The listing builds one solid part. Answer for the finished solid, in the listing's coordinates (mm). Face numbers are marked on the shaded views. A direction names the side the tool comes from. Round coordinates to 2 decimals unless told otherwise and drop trailing zeros. Loops run counter-clockwise (first coordinate to the right, second up) from the corner with the lowest first, then second, coordinate; pieces in that order, holes last. Notation, with made-up numbers: (-24.75, 5.25) -> (12.25, 5.25) arc R38 ccw to (12.25, 43.25) -> close; hole circle Ø6 at (47, -35). An arc over 180 degrees is marked (long way). One line per question, with ' | ' between items.
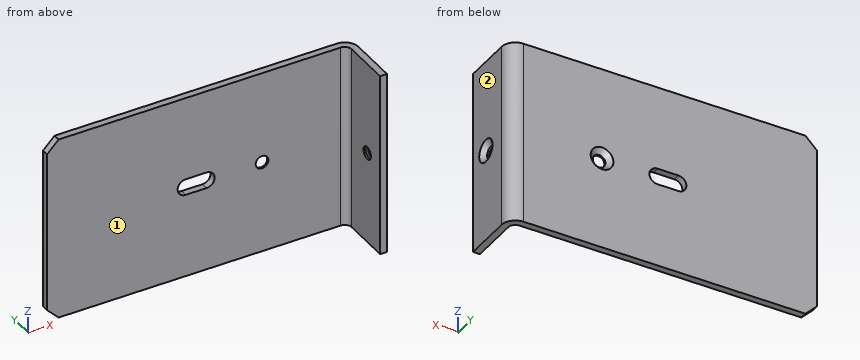
from build123d import *

# Parameters (mm, degrees)
BASE_EXTRU_MINCE_DEPTH  = 40
CHANFREIN1_SIZE         = 5
ESQUISSE3_R             = 2.75
ENL_V_MAT_EXTRU_1_DEPTH = 139.668669857
ESQUISSE4_R             = 2.75
ENL_V_MAT_EXTRU_2_DEPTH = 141.943250991
CHANFREIN2_SIZE         = 2.15


with BuildPart() as part:
    # Esquisse1 → Base-Extru.-Mince (new, symmetric)
    with BuildSketch(Plane.XY):
        with BuildLine():
            Line((0, -24), (0, -3))
            ThreePointArc((0, -3), (-0.878679656, -0.878679656), (-3, 0))
            Line((-3, 0), (-130, 0))
            Line((-130, 0), (-130, 3))
            Line((-130, 3), (-3, 3))
            ThreePointArc((-3, 3), (1.242640687, 1.242640687), (3, -3))
            Line((3, -3), (3, -24))
            Line((3, -24), (0, -24))
        make_face()
    extrude(amount=BASE_EXTRU_MINCE_DEPTH, both=True)

    # Chanfrein1
    chanfrein1_edges = [part.edges().sort_by_distance(p)[0] for p in [
        (-130, 1.5, 40),
        (-130, 1.5, -40),
    ]]
    chamfer(chanfrein1_edges, length=CHANFREIN1_SIZE)

    # Esquisse3 → Enl_v. mat.-Extru.1 (cut, through all)
    with BuildSketch(Plane(origin=(0, 3, 0), x_dir=(-1, 0, 0), z_dir=(0, 1, 0))):
        with Locations((37, 0)):
            Circle(ESQUISSE3_R)
        with BuildLine():
            Line((70, 3.5), (61, 3.5))
            ThreePointArc((61, 3.5), (57.5, 0), (61, -3.5))
            Line((61, -3.5), (70, -3.5))
            ThreePointArc((70, -3.5), (73.5, 0), (70, 3.5))
        make_face()
    extrude(amount=-ENL_V_MAT_EXTRU_1_DEPTH, mode=Mode.SUBTRACT)

    # Esquisse4 → Enl_v. mat.-Extru.2 (cut, through all)
    with BuildSketch(Plane(origin=(3, 0, 0), x_dir=(0, 0, -1), z_dir=(1, 0, 0))):
        with Locations(Location((0, -14.5, 0), (0, 0, 90))):
            Circle(ESQUISSE4_R)
    extrude(amount=-ENL_V_MAT_EXTRU_2_DEPTH, mode=Mode.SUBTRACT)

    # Chanfrein2
    chanfrein2_edges = [part.edges().sort_by_distance(p)[0] for p in [
        (-34.25, 3, 0),
        (3, -17.25, 0),
    ]]
    chamfer(chanfrein2_edges, length=CHANFREIN2_SIZE)


solid = part.part
Q1. For the marked faces 1 and 2, determine the directions among +Z, -Z, +X, -X, +Y, -Y from which every point of the face is accessible in a straight line to the end or side of a thin tool.
Numbers:
face 1: +Z, -Z, -X, -Y | face 2: +Z, -Z, +X, +Y, -Y
Q2. Find the intervals of material crossed by line 1 (Z direction, x = 0.7, y = -14.5); line 2 (Y direction, x = -69.5, z = -20), in increasing order. Write a range as from..to.
Numbers:
line 1: -40..-2.75, 2.75..40 | line 2: 0..3
Q3. A cutting plane is placed at D-D on x = -79. Give the vertices of the cut face in (y, z).
Numbers:
outline: (0, -40) -> (3, -40) -> (3, 40) -> (0, 40) -> close
Q4. A cutting plane is placed at C-C on z = 15. Give the vertices of the cut face in (x, y).
Numbers:
outline: (-130, 0) -> (-3, 0) arc R3 cw to (0, -3) -> (0, -24) -> (3, -24) -> (3, -3) arc R6 ccw to (-3, 3) -> (-130, 3) -> close
Q5. A cutting plane is placed at A-A on y = -14.5. Give the vertices of the cut face in (x, z), plus the area to 3 significant figures.
Numbers:
outline: (0, -40) -> (3, -40) -> (3, -4.9) -> (0.85, -2.75) -> (0, -2.75) -> close; (0, 2.75) -> (0.85, 2.75) -> (3, 4.9) -> (3, 40) -> (0, 40) -> close | area: 219 mm^2
Q6. Given pin 1 Ø2 at (y, z) = (-6, -19.5) entering from -X; pin 2 Ø6 at (x, z) = (-32.5, 25.5) entering from -Y; pin 3 Ø5 at (x, z) = (-37, 0) entering from -Y; pin 4 Ø6.5 at (y, z) = (-14.5, 0) entering from +X, each flat-ended and moving along its own axis, determine where each tip first touches the part or whether it passes through.
Numbers:
pin 1: x = 0 | pin 2: y = 0 | pin 3: through | pin 4: x = 1.35
